The model under review builds one solid part; all positions refer to its coordinate system, in mm. A direction names the side the tool comes from. Coordinates: 2 decimals unless noted, no trailing zeros. Loops run counter-clockwise (first coordinate to the right, second up) from the corner with the lowest first, then second, coordinate; pieces in that order, holes last. Notation, with made-up numbers: (-38, 81) - (-14, 81) arc R22 cw to (-14, 118) - close; hole circle Ø4 at (47.25, 26.25). An arc over 180 degrees is marked (long way). Use a Markdown table: item, result. Add a question column.
1) Clearance check with flat-ended pins moving along their axes: pin 1 (18 mm diameter, centred on y = -3, z = 38, fed in from -X); pin 2 (22.5 mm diameter, centred on x = 90, y = 9.5, fed in from +Z); pin 3 (12 mm diameter, centred on x = 14.5, z = -11, fed in from -Y); pin 4 (3 mm diameter, centred on y = 2.5, z = 7.5, fed in from -X). State where each tip first meets the part, or that it passes through.
2) Add section D-D, the plane z = 22. Give the boundary of the cut face in (x, y), and give its area (3 significant figures).
3) Add section B-B, the plane z = 71. Give the boundary of the cut face in (x, y).
4) For faces 4 (the flat face through (80, -10, 5)), 5 (the cylindrical face through (-185.282, -24.79, 76.737)), 6 (the flat face through (79.7, 10.3, 10.822)), 7 (the cylindrical face through (-36.61, -66.99, 57.15)), 8 (the flat face through (-150, 25, 30)), list the 3-axis set-ups (+Z, -Z, +X, -X, +Y, -Y) from which the entire face can be reached by the end or side of a thin tool; tool diameter is ignored.
5) Add section C-C, the plane x = -236. Give the boundary of the cut face in (y, z).
6) The part is to be moulded in two halves that separate along Y. For faces 1 (the flat face through (-212, -10, -18)), 2 (the cylindrical face through (57.52, 0.99, 35.76)), 3 (the flat face through (-7, 41, 0)), say which applies: pulls with the +Y half, pulls with the -Y half, needs draft (parallel to the pull), parting line crosses it, or undercut.
7) To check wall thickness, follow L1, parallel to X at y = -20, z = 37; L2, parallel to X at y = 17, z = 7; L3, parallel to X at y = -26, z = 13. State the ranges of each line that lie inside material, in increasing order. Write a range as [from, to].
8) Add section A-A, the plane x = 26.5. Give the boundary of the cut face in (y, z), and give its area (3 significant figures).
```python
from build123d import *

# Parameters (mm, degrees)
SKETCH_1_W               = 300
SKETCH_1_H               = 140
EXTRUDE_1_DEPTH          = 60
CUT_EXTRUDE_1_DEPTH      = 60
SKETCH_4_W               = 160
SKETCH_4_H               = 80
CUT_EXTRUDE_2_DEPTH      = 177.068168617
SKETCH_5_W               = 20
SKETCH_5_H               = 20
CUT_EXTRUDE_3_DEPTH      = 177.068168617
SKETCH_12_W              = 140
SKETCH_12_H              = 30
EXTRUDE_2_DEPTH          = 200
SKETCH_13_W              = 100
SKETCH_13_H              = 140
EXTRUDE_3_DEPTH          = 30
SKETCH_14_R              = 49
CUT_EXTRUDE_4_DEPTH      = 30
CUT_EXTRUDE_5_DEPTH      = 30
FILLET_3_R               = 10
SKETCH_17_R              = 22.5
CUT_EXTRUDE_6_DEPTH      = 49.178012217
CUT_EXTRUDE_7_DEPTH      = 368.903136522
CUT_EXTRUDE_7_DEPTH_BACK = 50
SKETCH_18_R              = 1.5
CUT_EXTRUDE_8_DEPTH      = 384.405790254


with BuildPart() as part:
    # 草图1 → 凸台-拉伸1 (new body)
    with BuildSketch(Plane.XY):
        Rectangle(SKETCH_1_W, SKETCH_1_H)
    extrude(amount=EXTRUDE_1_DEPTH)

    # 草图2 → 切除-拉伸1 (cut)
    with BuildSketch(Plane.XY.offset(60)):
        with BuildLine():
            Line((150, 0), (150, 70))
            Line((150, 70), (80, 70))
            ThreePointArc((80, 70), (129.497474683, 49.497474683), (150, 0))
        make_face()
        with BuildLine():
            Line((80, -70), (150, -70))
            Line((150, -70), (129.497474683, -49.497474683))
            ThreePointArc((129.497474683, -49.497474683), (106.787840266, -64.671567276), (80, -70))
        make_face()
        with BuildLine():
            Line((150, -70), (150, 0))
            ThreePointArc((150, 0), (144.671567276, -26.787840266), (129.497474683, -49.497474683))
            Line((129.497474683, -49.497474683), (150, -70))
        make_face()
    extrude(amount=-CUT_EXTRUDE_1_DEPTH, mode=Mode.SUBTRACT)

    # 草图4 → 切除-拉伸2 (cut, through all)
    with BuildSketch(Plane.XY.offset(60)):
        with Locations((-40, 0)):
            Rectangle(SKETCH_4_W, SKETCH_4_H)
    extrude(amount=-CUT_EXTRUDE_2_DEPTH, mode=Mode.SUBTRACT)

    # 草图5 → 切除-拉伸3 (cut, through all)
    with BuildSketch(Plane(origin=(0, 0, 0), x_dir=(-1, 0, 0), z_dir=(0, 0, -1))):
        with Locations((-80, 0)):
            Rectangle(SKETCH_5_W, SKETCH_5_H)
    extrude(amount=-CUT_EXTRUDE_3_DEPTH, mode=Mode.SUBTRACT)

    # 草图12 → 凸台-拉伸2 (add)
    with BuildSketch(Plane.ZY.offset(150)):
        with Locations((30, -55)):
            Rectangle(SKETCH_12_W, SKETCH_12_H)
    extrude(amount=EXTRUDE_2_DEPTH)

    # 草图13 → 凸台-拉伸3 (add)
    with BuildSketch(Plane(origin=(0, -40, 0), x_dir=(1, 0, 0), z_dir=(0, 1, 0))):
        with Locations((-200, -30)):
            Rectangle(SKETCH_13_W, SKETCH_13_H)
    extrude(amount=EXTRUDE_3_DEPTH)

    # 草图14 → 切除-拉伸4 (cut)
    with BuildSketch(Plane(origin=(0, -10, 0), x_dir=(1, 0, 0), z_dir=(0, 1, 0))):
        with Locations(Location((-200, -30, 0), (0, 0, 270))):
            Circle(SKETCH_14_R)
    extrude(amount=-CUT_EXTRUDE_4_DEPTH, mode=Mode.SUBTRACT)

    # 草图15 → 切除-拉伸5 (cut)
    with BuildSketch(Plane(origin=(0, -40, 0), x_dir=(1, 0, 0), z_dir=(0, 1, 0))):
        with BuildLine():
            ThreePointArc((-336, -50), (-337.171572875, -47.171572875), (-340, -46))
            Line((-340, -46), (-340, -54))
            ThreePointArc((-340, -54), (-337.171572875, -52.828427125), (-336, -50))
        make_face()
        with BuildLine():
            Line((-340, -54), (-340, -46))
            ThreePointArc((-340, -46), (-344, -50), (-340, -54))
        make_face()
        with BuildLine():
            ThreePointArc((-336, -10), (-337.171572875, -7.171572875), (-340, -6))
            Line((-340, -6), (-340, -14))
            ThreePointArc((-340, -14), (-337.171572875, -12.828427125), (-336, -10))
        make_face()
        with BuildLine():
            Line((-340, -14), (-340, -6))
            ThreePointArc((-340, -6), (-344, -10), (-340, -14))
        make_face()
    extrude(amount=-CUT_EXTRUDE_5_DEPTH, mode=Mode.SUBTRACT)

    # 圆角3
    fillet_3_edges = [part.edges().sort_by_distance(p)[0] for p in [
        (-35, 70, 0),
        (-35, 70, 60),
        (-35, -70, 60),
        (150, 0, 60),
        (150, 0, 0),
        (-35, -70, 0),
        (-150, 70, 30),
    ]]
    fillet(fillet_3_edges, radius=FILLET_3_R)

    # 草图17 → 切除-拉伸6 (cut)
    with BuildSketch(Plane.XY.offset(60)):
        with Locations((80, 0)):
            Circle(SKETCH_17_R)
    extrude(amount=-CUT_EXTRUDE_6_DEPTH, mode=Mode.SUBTRACT)

    # 草图18 → 切除-拉伸7 (cut, two sides: drawn at the far end of the back side and taken through both)
    with BuildSketch(Plane.XY.offset(10.821987783).offset(-CUT_EXTRUDE_7_DEPTH_BACK)):
        with Locations(Location((80, 17.5, 0), (0, 0, 180))):
            Circle(SKETCH_18_R)
        with Locations(Location((95.155444566, 8.75, 0), (0, 0, 180))):
            Circle(SKETCH_18_R)
        with Locations(Location((95.155444566, -8.75, 0), (0, 0, 180))):
            Circle(SKETCH_18_R)
        with Locations(Location((80, -17.5, 0), (0, 0, 180))):
            Circle(SKETCH_18_R)
        with Locations(Location((64.844555434, -8.75, 0), (0, 0, 180))):
            Circle(SKETCH_18_R)
        with Locations(Location((64.844555434, 8.75, 0), (0, 0, 180))):
            Circle(SKETCH_18_R)
    extrude(amount=CUT_EXTRUDE_7_DEPTH + CUT_EXTRUDE_7_DEPTH_BACK, mode=Mode.SUBTRACT)

    # 草图19 → 切除-拉伸8 (cut, through all)
    with BuildSketch(Plane.XY.offset(100)):
        with BuildLine():
            ThreePointArc((-196, -30), (-200, -26), (-204, -30))
            Line((-204, -30), (-196, -30))
        make_face()
        with BuildLine():
            Line((-196, -30), (-204, -30))
            ThreePointArc((-204, -30), (-200, -34), (-196, -30))
        make_face()
    extrude(amount=-CUT_EXTRUDE_8_DEPTH, mode=Mode.SUBTRACT)


solid = part.part
```
From the geometry:
| question | item | result |
|---|---|---|
| 1 | pin 1 | stops at x = -250 |
| 1 | pin 2 | stops at z = 60 |
| 1 | pin 3 | passes through |
| 1 | pin 4 | stops at x = -150 |
| 2 | outline | (-350, -70) - (80, -70) arc R70 ccw to (80, 70) - (-140, 70) arc R10 ccw to (-150, 60) - (-150, -10) - (-151.66, -10) - (-151.66, -40) - (-248.34, -40) - (-248.34, -10) - (-250, -10) - (-250, -40) - (-350, -40) - close; hole (-120, -40) - (40, -40) - (40, 40) - (-120, 40) - close; hole circle Ø45 at (80, 0) |
| 2 | area | 31,600 mm^2 |
| 3 | outline | (-350, -70) - (-150, -70) - (-150, -10) - (-173.17, -10) - (-173.17, -40) - (-226.83, -40) - (-226.83, -10) - (-250, -10) - (-250, -40) - (-350, -40) - close |
| 4 | face 4 | +Z, -Z |
| 4 | face 5 | +Y |
| 4 | face 6 | +Z |
| 4 | face 7 | +Z, +X, -Y |
| 4 | face 8 | +Z, -Z, -X, +Y |
| 5 | outline | (-70, -40) - (-10, -40) - (-10, -3.24) - (-40, -3.24) - (-40, 63.24) - (-10, 63.24) - (-10, 100) - (-70, 100) - close |
| 6 | face 1 | pulls with the +Y half |
| 6 | face 2 | undercut |
| 6 | face 3 | needs draft |
| 7 | L1 | x = [-250, -248.5], [-151.5, -120], [40, 69.69], [90.31, 147.08] |
| 7 | L2 | x = [-150, -120], [40, 78.59], [81.41, 147.43] |
| 7 | L3 | x = [-250, -245.96], [-154.04, -120], [40, 144.99] |
| 8 | outline | (-70, 10) arc R10 ccw to (-60, 0) - (-40, 0) - (-40, 60) - (-60, 60) arc R10 ccw to (-70, 50) - close; (40, 0) - (60, 0) arc R10 ccw to (70, 10) - (70, 50) arc R10 ccw to (60, 60) - (40, 60) - close |
| 8 | area | 3,510 mm^2 |
